Here's how the part is built. I have some questions about the finished solid (model axes, mm). Face numbers are marked on the shaded views. A direction names the side the tool comes from. Coordinates: 2 decimals unless noted, no trailing zeros. Write each loop counter-clockwise with the first axis right and the second up, starting at its lowest first coordinate (ties: lowest second). Pieces come first, ordered by that corner, then holes. Notation, with made-up numbers: (-9, 28.25) -> (49, 28.25) arc R4 ccw to (49, 33.25) -> close; hole circle Ø7 at (32, -25). An arc over 180 degrees is marked (long way). Put each result on its own line as item: value.
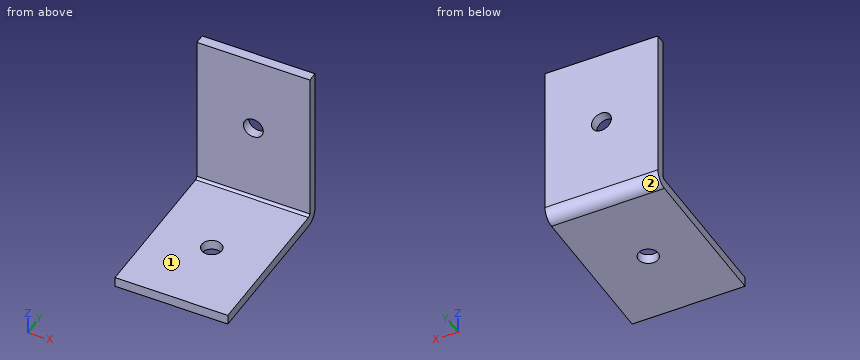
```python
from build123d import *

# Parameters (mm, degrees)
SKETCH1_W                    = 34
SKETCH1_H                    = 3
BASE_FLANGE1_DEPTH           = 50
EDGE_FLANGE1_STRIP_W         = 13.4732
EDGE_FLANGE1_STRIP_H         = 3
EDGE_FLANGE1_STRIP_CUT_DEPTH = 34
EDGE_FLANGE1_DEPTH           = 34
SKETCH9_R                    = 3
CUT_EXTRUDE1_DEPTH           = 10
SKETCH10_R                   = 3
CUT_EXTRUDE2_DEPTH           = 10


# Sheet-metal steps are written as plain solids
with BuildPart() as part:
    # Sketch1 → Base-Flange1 (new body)
    with BuildSketch(Plane(origin=(0, 0, 0), x_dir=(1, 0, 0), z_dir=(0, 1, 0))):
        with Locations((17, -1.5)):
            Rectangle(SKETCH1_W, SKETCH1_H)
    extrude(amount=BASE_FLANGE1_DEPTH)

    # Edge-Flange1 strip (across the edge) → Edge-Flange1 strip cut (cut)
    with BuildSketch(Plane(origin=(34, 50, 3), x_dir=(0, -1, 0), z_dir=(-1, 0, 0))):
        with Locations((-3, -1.5)):
            Rectangle(EDGE_FLANGE1_STRIP_W, EDGE_FLANGE1_STRIP_H)
    extrude(amount=EDGE_FLANGE1_STRIP_CUT_DEPTH, mode=Mode.SUBTRACT)

    # Edge-Flange1 section (across the edge) → Edge-Flange1 (add)
    with BuildSketch(Plane(origin=(34, 50, 3), x_dir=(0, -1, 0), z_dir=(-1, 0, 0))):
        with BuildLine():
            Line((0, 0.7366), (0, 47))
            Line((0, 47), (3, 47))
            Line((3, 47), (3, 0.7366))
            ThreePointArc((3, 0.7366), (3.215745145, 0.215745145), (3.7366, 0))
            Line((3.7366, 0), (3.7366, -3))
            ThreePointArc((3.7366, -3), (1.094424801, -1.905575199), (0, 0.7366))
        make_face()
    extrude(amount=EDGE_FLANGE1_DEPTH)

    # Sketch9 → Cut-Extrude1 (cut)
    with BuildSketch(Plane(origin=(0, 50, 0), x_dir=(1, 0, 0), z_dir=(0, 1, 0))):
        with Locations(Location((17, -26.8683, 0), (0, 0, 270))):
            Circle(SKETCH9_R)
    extrude(amount=-CUT_EXTRUDE1_DEPTH, mode=Mode.SUBTRACT)

    # Sketch10 → Cut-Extrude2 (cut)
    with BuildSketch(Plane.XY.offset(3)):
        with Locations((17, 23.1317)):
            Circle(SKETCH10_R)
    extrude(amount=-CUT_EXTRUDE2_DEPTH, mode=Mode.SUBTRACT)


solid = part.part
```
Item 1: Which directions (+Z, -Z, +X, -X, +Y, -Y) give clear straight access to the entire face, cutting with the end or side of a thin tool? Please do the marked faces 1 and 2.
Output:
face 1: +Z, +X, -X, -Y
face 2: -Z, +X, -X, +Y
Item 2: Please list where these lines run through material, in increasing order: line 1 along Y through (x, z) = (12.5, 8.5); line 2 along Z through (x, y) = (10.5, 12); line 3 along Y through (x, z) = (17, 0.95). Write a range as from..to.
Output:
line 1: y = 47..50
line 2: z = 0..3
line 3: y = 0..20.13, 26.13..48.75
Item 3: Imagine slicing it at B-B on x = 26. Write out the boundary of the cut face in (y, z), then the cut area to 3 significant figures.
Output:
outline: (0, 0) -> (46.26, 0) arc R3.74 ccw to (50, 3.74) -> (50, 50) -> (47, 50) -> (47, 3.74) arc R0.74 cw to (46.26, 3) -> (0, 3) -> close
area: 288 mm²
Item 4: Imagine slicing it at A-A on x = 17. Write out the boundary of the cut face in (y, z).
Output:
outline: (0, 0) -> (20.13, 0) -> (20.13, 3) -> (0, 3) -> close; (26.13, 0) -> (46.26, 0) arc R3.74 ccw to (50, 3.74) -> (50, 23.87) -> (47, 23.87) -> (47, 3.74) arc R0.74 cw to (46.26, 3) -> (26.13, 3) -> close; (47, 29.87) -> (50, 29.87) -> (50, 50) -> (47, 50) -> close
Item 5: Imagine slicing it at C-C on z = 19. Write out the boundary of the cut face in (x, y).
Output:
outline: (0, 47) -> (34, 47) -> (34, 50) -> (0, 50) -> close
Item 6: Imagine slicing it at D-D on y = 30. Write out the boundary of the cut face in (x, z), then the cut area to 3 significant figures.
Output:
outline: (0, 0) -> (34, 0) -> (34, 3) -> (0, 3) -> close
area: 102 mm²
Item 7: For P1, Ø17, axis at x = 20.5, z = 25.5, coming from the -Y side; P2, Ø8, axis at x = 17, z = 26.87, coming from the +Y side; P3, Ø4, axis at x = 17.5, y = 43, coming from the +Z side, each with a flat end and sliding along its axis, tell me the tip position at first contact or that it passes through.
Output:
P1: stops at y = 47
P2: stops at y = 50
P3: stops at z = 3
